Can you work these out from the model? Positions are in its coordinate system, mm. Face numbers are marked on the shaded views. A direction names the side the tool comes from. Give positions to 0.01 mm unless a question says otherwise; leave off trailing zeros. Write each loop counter-clockwise with the first axis right and the second up, starting at its lowest first coordinate (ties: lowest second). Pieces come first, ordered by that corner, then holes.
from build123d import *

# Parameters (mm, degrees)
F1_DEPTH  = 47.5
F2_R      = 44.99999
F3_R      = 5
F4_R      = 18.5
F5_DEPTH  = 95.001
F4_R_2    = 25
F6_DEPTH  = 22
F8_DEPTH  = 20.001
F7_R      = 12.5
F7_R_2    = 7
F9_DEPTH  = 6
F10_DEPTH = 20.001


# Not quite as in the source:
# - a fillet or chamfer is up to 0.001 mm smaller than in the source, because OpenCascade refuses the exact size
# - a pattern or mirror of a feature is missing from the dataset's text; its kind, count and spacing are read off the source's solid


with BuildPart() as f1:
    # F0 (on Front) → F1 (new body, symmetric)
    with BuildSketch(Plane.XZ):
        Polygon((-45, 10), (-125, 10), (-125, -10), (125, -10), (125, 10), (45, 10), (45, 90), (-45, 90), align=None)
    extrude(amount=F1_DEPTH, both=True)

    # F2 (radius 45 in the source; OpenCascade refuses exactly that, so slightly less here)
    f2_edges = [f1.edges().sort_by_distance(p)[0] for p in [
        (45, 0, 90),
        (-45, 0, 90),
    ]]
    fillet(f2_edges, radius=F2_R)

    # F3
    f3_edges = [f1.edges().sort_by_distance(p)[0] for p in [
        (45, 0, 10),
        (-45, 0, 10),
    ]]
    fillet(f3_edges, radius=F3_R)

    # F4 (on face) → F5 (cut, through all)
    with BuildSketch(Plane.XZ.offset(47.5)):
        with Locations((0, 45)):
            Circle(F4_R)
    extrude(amount=-F5_DEPTH, mode=Mode.SUBTRACT)

    # F4 (on face) → F6 (cut)
    with BuildSketch(Plane.XZ.offset(47.5)):
        with Locations((0, 45)):
            Circle(F4_R_2)
        with Locations((0, 45)):
            Circle(F4_R, mode=Mode.SUBTRACT)
    extrude(amount=-F6_DEPTH, mode=Mode.SUBTRACT)

    # F7 (on face) → F8 (cut, through all)
    with BuildSketch(Plane.XY.offset(10)):
        with BuildLine():
            Line((125, -15), (125, 15))
            Line((125, 15), (107, 15))
            ThreePointArc((107, 15), (92, 0), (107, -15))
            Line((107, -15), (125, -15))
        make_face()
    f8 = extrude(amount=-F8_DEPTH, mode=Mode.SUBTRACT)

    # F8_copies: F8 across plane
    add(f8.mirror(Plane(origin=(0, 0, 0), x_dir=(0, 0, -1), z_dir=(-1, 0, 0))), mode=Mode.SUBTRACT)

    # F7 (on face) → F9 (cut)
    with BuildSketch(Plane.XY.offset(10)):
        with Locations((75, 25)):
            Circle(F7_R)
        with Locations((75, 25)):
            Circle(F7_R_2, mode=Mode.SUBTRACT)
    f9 = extrude(amount=-F9_DEPTH, mode=Mode.SUBTRACT)

    # F9_copies: F9 across plane
    add(f9.mirror(Plane(origin=(0, 0, 0), x_dir=(0, 0, -1), z_dir=(-1, 0, 0))), mode=Mode.SUBTRACT)

    # F9_copies1: F9 across plane
    add(f9.mirror(Plane(origin=(0, 0, 0), x_dir=(0, 0, -1), z_dir=(0, -1, 0))), mode=Mode.SUBTRACT)

    # F9_copies2: F9 across plane
    add(f9.mirror(Plane(origin=(0, 0, 0), x_dir=(0.316227766, -0.9486832981, 0), z_dir=(-0.9486832981, -0.316227766, 0))), mode=Mode.SUBTRACT)

    # F7 (on face) → F10 (cut, through all)
    with BuildSketch(Plane.XY.offset(10)):
        with Locations((75, 25)):
            Circle(F7_R_2)
    f10 = extrude(amount=-F10_DEPTH, mode=Mode.SUBTRACT)

    # F10_copies: F10 across plane
    add(f10.mirror(Plane(origin=(0, 0, 0), x_dir=(0, 0, -1), z_dir=(0, -1, 0))), mode=Mode.SUBTRACT)

    # F10_copies1: F10 across plane
    add(f10.mirror(Plane(origin=(0, 0, 0), x_dir=(0, 0, -1), z_dir=(-1, 0, 0))), mode=Mode.SUBTRACT)

    # F10_copies2: F10 across plane
    add(f10.mirror(Plane(origin=(0, 0, 0), x_dir=(0.316227766, -0.9486832981, 0), z_dir=(-0.9486832981, -0.316227766, 0))), mode=Mode.SUBTRACT)


solid = f1.part
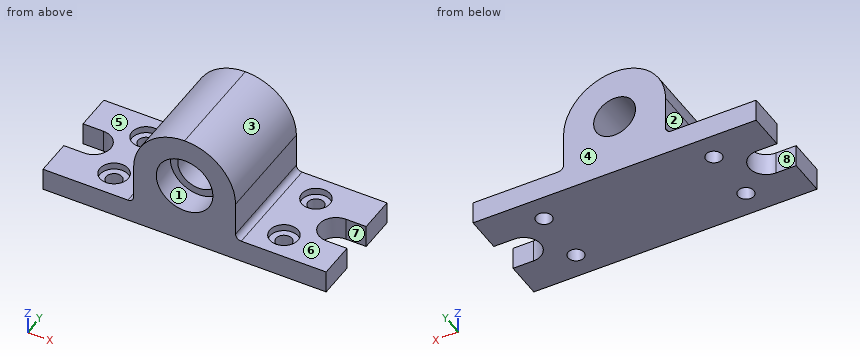
(1) If we mould it in two halves opening along Z, with no side actions, what happens to the marked faces 1, 2 and 3? For each: +Z half, -Z half, draft (parallel to the pull), parting line (faces both ways), or undercut.
Returned:
face 1: undercut
face 2: draft
face 3: +Z half
(2) Imagine slicing it at D-D, the plane z = 59. Write out the boundary of the cut face in (x, y), plus the area to 3 significant figures.
Returned:
outline: (-42.77, -47.5) - (-20.71, -47.5) - (-20.71, -25.5) - (-12.09, -25.5) - (-12.09, 47.5) - (-42.77, 47.5) - close; (12.09, -25.5) - (20.71, -25.5) - (20.71, -47.5) - (42.77, -47.5) - (42.77, 47.5) - (12.09, 47.5) - close
area: 5,450 mm2
(3) Imagine slicing it at A-A, the plane y = 25. Give the number of separate pieces and of enclosed holes in the cut face, plus the area to 3 significant figures.
Returned:
separate pieces: 3
enclosed holes: 1
area: 9,570 mm2
(4) Imagine slicing it at B-B, the plane x = 75. Write out the boundary of the cut face in (y, z), plus the area to 3 significant figures.
Returned:
outline: (-47.5, -10) - (-32, -10) - (-32, 4) - (-37.5, 4) - (-37.5, 10) - (-47.5, 10) - close; (-18, -10) - (18, -10) - (18, 4) - (12.5, 4) - (12.5, 10) - (-12.5, 10) - (-12.5, 4) - (-18, 4) - close; (32, -10) - (47.5, -10) - (47.5, 10) - (37.5, 10) - (37.5, 4) - (32, 4) - close
area: 1,210 mm2
(5) If I drill on L1, parallel to Y at x = 75, z = 5.7; L2, parallel to Y at x = 75, z = -2.75; L3, parallel to X at y = -25, z = -1.25, over which ranges is the centre line in solid material (lowest first)?
Returned:
L1: y = -47.5 to -37.5, -12.5 to 12.5, 37.5 to 47.5
L2: y = -47.5 to -32, -18 to 18, 32 to 47.5
L3: x = -125 to -82, -68 to 68, 82 to 125
(6) For the marked faces 4, 5, 6, 7 and 8, which set-ups out of +Z, -Z, +X, -X, +Y, -Y let a thin tool reach every point of the face, with its end or its side?
Returned:
face 4: +Z, -Z, +X, -X, +Y
face 5: +Z, -X, +Y, -Y
face 6: +Z, +X, +Y, -Y
face 7: +Z, -Z, +X
face 8: +Z, -Z, -X
(7) Will these pins go through, and if not, where does the flat tip stop? P1, Ø12.5, axis at x = 75, y = -25, coming from the -Z side; P2, Ø6, axis at x = 76, y = 8, coming from the +Z side; P3, Ø5, axis at y = -23.5, z = 22, coming from the -X side; P4, Ø1, axis at y = 26, z = 72.5, coming from the +X side.
Returned:
P1: passes through
P2: stops at z = 10
P3: stops at x = -45
P4: stops at x = 36
